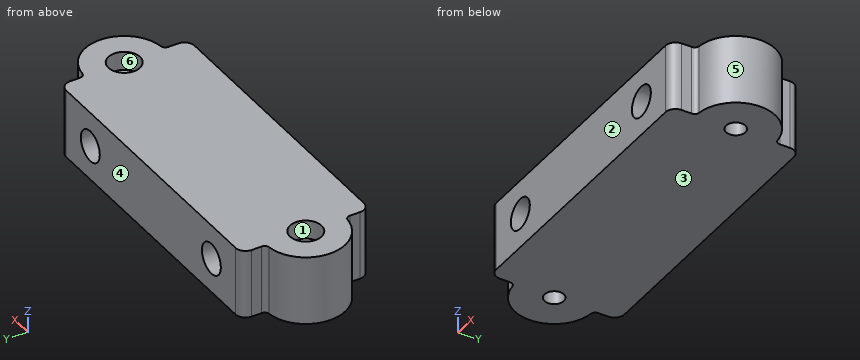
from build123d import *

# Parameters (mm, degrees)
SKETCH1_W           = 101.6
SKETCH1_H           = 17.78
SKETCH1_R           = 3.96875
BOSS_EXTRUDE1_DEPTH = 33.02
SKETCH2_R           = 2.4892
CUT_EXTRUDE1_DEPTH  = 17.78
SKETCH3_R           = 4.064
CUT_EXTRUDE2_DEPTH  = 4.826
CUT_EXTRUDE3_DEPTH  = 109.300548475
FILLET1_R           = 2.54


with BuildPart() as part:
    # Sketch1 → Boss-Extrude1 (new body)
    with BuildSketch(Plane(origin=(0, 0, 0), x_dir=(1, 0, 0), z_dir=(0, 1, 0))):
        with Locations((50.8, 8.89)):
            Rectangle(SKETCH1_W, SKETCH1_H)
        with Locations(Location((76.2, 8.89, 0), (0, 0, 270))):
            Circle(SKETCH1_R, mode=Mode.SUBTRACT)
        with Locations(Location((25.4, 8.89, 0), (0, 0, 270))):
            Circle(SKETCH1_R, mode=Mode.SUBTRACT)
    extrude(amount=-BOSS_EXTRUDE1_DEPTH)

    # Sketch2 → Cut-Extrude1 (cut)
    with BuildSketch(Plane.XY):
        with Locations((88.9, -16.51)):
            Circle(SKETCH2_R)
        with Locations((12.7, -16.51)):
            Circle(SKETCH2_R)
    extrude(amount=-CUT_EXTRUDE1_DEPTH, mode=Mode.SUBTRACT)

    # Sketch3 → Cut-Extrude2 (cut)
    with BuildSketch(Plane.XY):
        with Locations((88.9, -16.51)):
            Circle(SKETCH3_R)
        with Locations((12.7, -16.51)):
            Circle(SKETCH3_R)
    extrude(amount=-CUT_EXTRUDE2_DEPTH, mode=Mode.SUBTRACT)

    # Sketch5 → Cut-Extrude3 (cut, through all)
    with BuildSketch(Plane.XY):
        with BuildLine():
            Line((12.7, -5.150774674), (12.7, 0))
            Line((12.7, 0), (0, 0))
            Line((0, 0), (0, -33.02))
            Line((0, -33.02), (12.7, -33.02))
            Line((12.7, -33.02), (12.7, -27.869225326))
            ThreePointArc((12.7, -27.869225326), (12.37660211, -27.022558659), (11.571111111, -26.607089178))
            ThreePointArc((11.571111111, -26.607089178), (2.54, -16.51), (11.571111111, -6.412910822))
            ThreePointArc((11.571111111, -6.412910822), (12.37660211, -5.997441341), (12.7, -5.150774674))
        make_face()
        with BuildLine():
            Line((88.9, -5.150774674), (88.9, 0))
            Line((88.9, 0), (101.6, 0))
            Line((101.6, 0), (101.6, -33.02))
            Line((101.6, -33.02), (88.9, -33.02))
            Line((88.9, -33.02), (88.9, -27.869225326))
            ThreePointArc((88.9, -27.869225326), (89.22339789, -27.022558659), (90.028888889, -26.607089178))
            ThreePointArc((90.028888889, -26.607089178), (99.06, -16.51), (90.028888889, -6.412910822))
            ThreePointArc((90.028888889, -6.412910822), (89.22339789, -5.997441341), (88.9, -5.150774674))
        make_face()
    extrude(amount=-CUT_EXTRUDE3_DEPTH, mode=Mode.SUBTRACT)

    # Fillet1
    fillet1_edges = [part.edges().sort_by_distance(p)[0] for p in [
        (12.7, -33.02, -8.89),
        (12.7, 0, -8.89),
        (88.9, 0, -8.89),
        (88.9, -33.02, -8.89),
    ]]
    fillet(fillet1_edges, radius=FILLET1_R)


solid = part.part
Read the model definition and answer for the solid it produces. Units are mm, in the model's axes. Face numbers are marked on the shaded views. A direction names the side the tool comes from. Coordinates: 2 decimals unless noted, no trailing zeros. Write each loop counter-clockwise with the first axis right and the second up, starting at its lowest first coordinate (ties: lowest second). Pieces come first, ordered by that corner, then holes. Notation, with made-up numbers: (85.25, -40) -> (140.25, -40) arc R14 ccw to (140.25, -22) -> close; hole circle Ø4 at (-14.5, 17). An arc over 180 degrees is marked (long way). Return JSON: item names as keys, results as strings.
(1) The part is cut by section C-C on z = -3. Give the vertices of the cut face in (x, y).
Answers below:
{"outline": "(11.57, -26.61) arc R1.27 cw to (12.7, -27.87) -> (12.7, -30.48) arc R2.54 ccw to (15.24, -33.02) -> (86.36, -33.02) arc R2.54 ccw to (88.9, -30.48) -> (88.9, -27.87) arc R1.27 cw to (90.03, -26.61) arc R10.16 ccw to (90.03, -6.41) arc R1.27 cw to (88.9, -5.15) -> (88.9, -2.54) arc R2.54 ccw to (86.36, 0) -> (15.24, 0) arc R2.54 ccw to (12.7, -2.54) -> (12.7, -5.15) arc R1.27 cw to (11.57, -6.41) arc R10.16 ccw to start; hole circle Ø8.13 at (12.7, -16.51); hole circle Ø8.13 at (88.9, -16.51)"}
(2) The part is cut by section A-A on z = -8.89. Give the vertices of the cut face in (x, y).
Answers below:
{"outline": "(11.57, -26.61) arc R1.27 cw to (12.7, -27.87) -> (12.7, -30.48) arc R2.54 ccw to (15.24, -33.02) -> (21.43, -33.02) -> (21.43, 0) -> (15.24, 0) arc R2.54 ccw to (12.7, -2.54) -> (12.7, -5.15) arc R1.27 cw to (11.57, -6.41) arc R10.16 ccw to start; (29.37, -33.02) -> (72.23, -33.02) -> (72.23, 0) -> (29.37, 0) -> close; (80.17, -33.02) -> (86.36, -33.02) arc R2.54 ccw to (88.9, -30.48) -> (88.9, -27.87) arc R1.27 cw to (90.03, -26.61) arc R10.16 ccw to (90.03, -6.41) arc R1.27 cw to (88.9, -5.15) -> (88.9, -2.54) arc R2.54 ccw to (86.36, 0) -> (80.17, 0) -> close; hole circle Ø4.98 at (12.7, -16.51); hole circle Ø4.98 at (88.9, -16.51)"}
(3) The part is cut by section D-D on y = -4. Give the vertices of the cut face in (x, z), then the cut area to 3 significant figures.
Answers below:
{"outline": "(12.7, -17.78) -> (88.9, -17.78) -> (88.9, 0) -> (12.7, 0) -> close; hole circle Ø7.94 at (25.4, -8.89); hole circle Ø7.94 at (76.2, -8.89)", "area": "1,260 mm^2"}
(4) Consider line 1 along X through (y, z) = (-4, -11.5); line 2 along Z through (x, y) = (25, -23); line 3 along X through (y, z) = (-25, -8.89). Determine where each line is inside the solid, lowest interval first. Write a range as from..to.
Answers below:
{"line 1": "12.7..22.41, 28.39..73.21, 79.19..88.9", "line 2": "-17.78..-12.84, -4.94..0", "line 3": "7.12..21.43, 29.37..72.23, 80.17..94.48"}
(5) Each of these flat-tipped pins is pushed along its axis until it touches: P1, Ø3, axis at y = -14, z = -4.5, coming from the -X side; P2, Ø6.5, axis at x = 76.2, z = -8.89, coming from the +Y side; P3, Ø4, axis at x = 90, y = -16, coming from the +Z side; P4, Ø1.3, axis at y = -29, z = -12.5, coming from the -X side. Where does it stop, or does it pass through?
Answers below:
{"P1": "x = 2.59", "P2": "through", "P3": "z = -4.83", "P4": "x = 12.7"}
(6) The part is cut by section B-B on x = 25.4. Give the vertices of the cut face in (y, z).
Answers below:
{"outline": "(-33.02, -17.78) -> (0, -17.78) -> (0, -12.86) -> (-33.02, -12.86) -> close; (-33.02, -4.92) -> (0, -4.92) -> (0, 0) -> (-33.02, 0) -> close"}
(7) For a pull along Y with two mould halves and no side action, classify the marked faces 1, 2, 3 and 4 as pulls with the +Y half, pulls with the -Y half, needs draft (parallel to the pull), parting line crosses it, or undercut.
Answers below:
{"face 1": "undercut", "face 2": "pulls with the -Y half", "face 3": "needs draft", "face 4": "pulls with the +Y half"}
(8) Which of the six approach directions +Z, -Z, +X, -X, +Y, -Y give full straight-line access (tool end or side, diameter ignored) to the marked faces 5 and 6?
Answers below:
{"face 5": "+Z, -Z, +X", "face 6": "+Z"}
